Autodesk Fusion 360 part; units mm, degrees
sketch "Sketch1" plane through (0, 0, 0) normal (0, 1, 0) x (1, 0, 0)
  line L0 (-24, 0) -> (24, 0)
  line L1 (1.75, 0) -> (22.5, 0)
  line L2 (0, -1.75) -> (0, -22.5)
  line L3 (-24, 0) -> (-24, -15)
  line L4 (-24, -15) -> (-16, -15)
  line L5 (-16, -15) -> (24, 0)
  dimension "d1" = 48
  dimension "d2" = 15
  dimension "d3" = 8
extrude "Extrude1" add sketch "Sketch1" along normal blind 28.2
ref_plane "WorkPlane1" through (0, 1.88, 7.5) normal (0, -1, 0) x (-1, 0, 0)
sketch "Sketch2" plane through (0, 1.88, 7.5) normal (0, -1, 0) x (1, 0, 0)
  line L0 (-16, 7.5) -> (24, -7.5)
  line L1 (24, -7.5) -> (-24, -7.5)
  line L2 (18.6667, -5.5) -> (-16, -5.5)
  line L3 (-16, -5.5) -> (-16, 7.5)
  line L4 (18.6667, 7.5) -> (-16, 7.5)
  line L5 (18.6667, -5.5) -> (18.6667, 7.5)
  dimension "d7" = 2
extrude "Extrude2" cut sketch "Sketch2" against normal blind 1.88
pattern_linear "R-Pattern1" count 7 spacing 3.76 along (0, 1, 0) of "Extrude2"
equation "d4 = ( ( 1.88 * 2 ) * 1 mm ) * 7 + 1.88 mm"
equation "d12 = -1.88 * 2 mm"
For this review, take the finished solid that the model builds, in its own axes (mm). A direction names the side the tool comes from. Round coordinates to 2 decimals unless told otherwise and drop trailing zeros. Write each loop counter-clockwise with the first axis right and the second up, starting at its lowest first coordinate (ties: lowest second). Pieces come first, ordered by that corner, then holes. Notation, with made-up numbers: M 73.25,-30.5 L 112.25,-30.5 A27 ccw 112.25,-6.5 Z; hole C 79,43 d2. An arc over 180 degrees is marked long. One line per item, written item: value. Start each with the question number.
(1) Machinability: for faces 1 (the flat face through (-20, 14, 15)), 2 (the flat face through (-7, 20.68, 6)), which of the approach directions +Z, -Z, +X, -X, +Y, -Y give a long, thin tool a straight path to every point of the face, cutting with its end or side? Answer none if there is none.
(2) We need section B-B (y = 7). Give the boundary of the cut face in (x, z), and give its area (3 significant figures).
(3) Insertion check: pin 1 (1.5 mm diameter, centred on y = 10.5, z = 6, fed in from +X); pin 2 (2 mm diameter, centred on x = 0, y = 13.5, fed in from +Z); pin 3 (10 mm diameter, centred on x = 8.5, y = 15, fed in from +Z); pin 4 (6.5 mm diameter, centred on x = -4, z = 11.5, fed in from +Y). Each pin has a flat end and moves straight along its axis. Give the tip position at first contact, or say it passes through.
(4) Wall thickness on line 1 (X direction, y = 3.25, z = 9.5); line 2 (Z direction, x = -8.5, y = 17); line 3 (Z direction, x = -12, y = 15.25): over which ranges is each line inside the solid? List them lowest first.
(5) The part is to be moulded in two halves that separate along Y. For faces 3 (the flat face through (-3, 9.4, 7)), 4 (the flat face through (-6, 28.2, 6)), 5 (the flat face through (0, 14, 0)), say which applies: released by +Y, released by -Y, zero draft, split by the parting line, or undercut.
Result:
1. face 1: +Z, +X, -X, +Y, -Y
1. face 2: +Z, +X
2. outline: M -24,0 L 24,0 L 18.67,2 L -16,2 L -16,15 L -24,15 Z
2. area: 195 mm²
3. pin 1: x = -16
3. pin 2: z = 9.35
3. pin 3: z = 7.69
3. pin 4: y = 28.2
4. line 1: -24 to -16
4. line 2: 0 to 2
4. line 3: 0 to 13.5
5. face 3: undercut
5. face 4: released by +Y
5. face 5: zero draft
